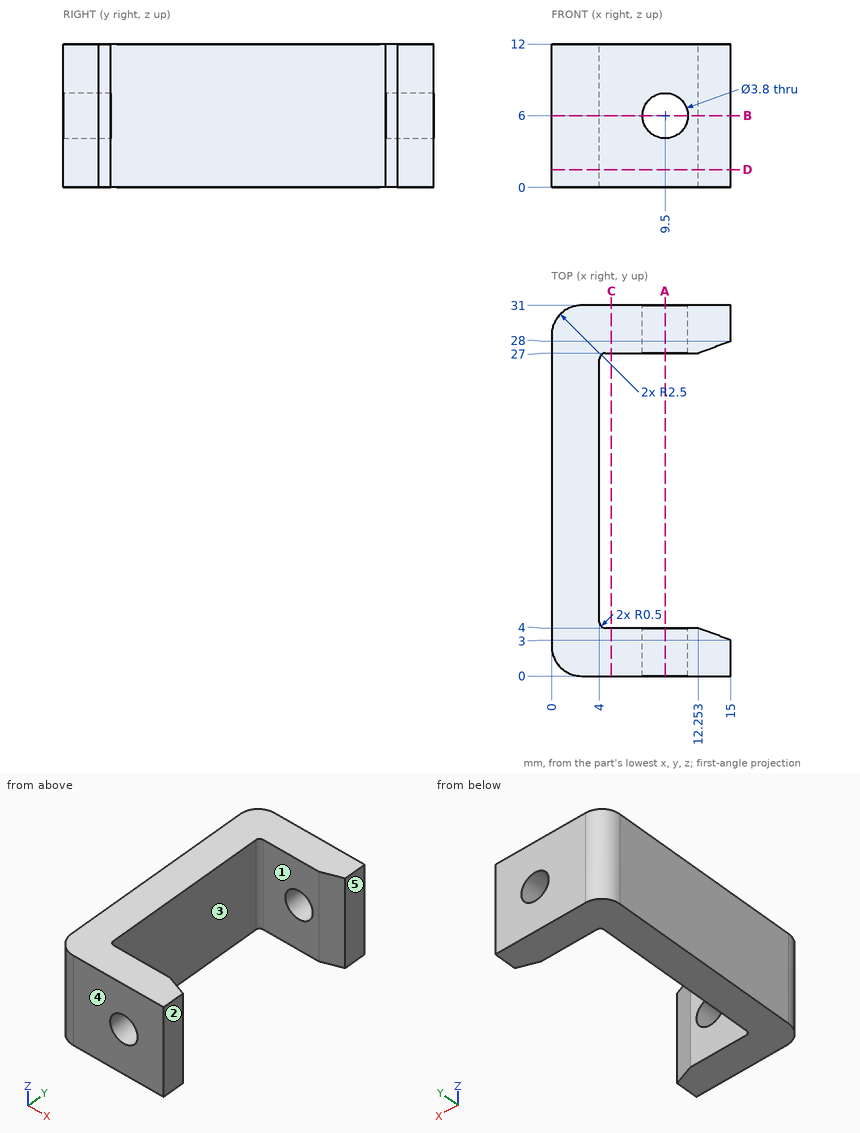
Check sheet for the drawn part. Datum: minimum x, y, z corner. Units: mm. A direction names the side the tool comes from. Round coordinates to 2 decimals unless told otherwise and drop trailing zeros. Order: outer loops, then holes, each group sorted by start corner. A loop starts at its lowest first (then second) coordinate and runs counter-clockwise, first axis right, second up. Notation, with made-up numbers: (10.5, 15) -> (38.5, 15) arc R37 cw to (38.5, 53) -> close; hole circle Ø9 at (53.5, -20). An arc over 180 degrees is marked (long way). Use CSV: the item, a comma, the result in double quotes.
(1) Cross-section at C-C (x = 5). Record the boundary of the cut face in (y, z).
Worked out:
outline,"(0, 0) -> (4, 0) -> (4, 12) -> (0, 12) -> close; (27, 0) -> (31, 0) -> (31, 12) -> (27, 12) -> close"
(2) Tool access check on the marked faces 1 and 2. Record the directions out of +Z, -Z, +X, -X, +Y, -Y that give a thin tool (end or side, any length) a straight path to the whole face; none if there is none.
Worked out:
face 1,"+Z, -Z, +X"
face 2,"+Z, -Z, +X, +Y, -Y"
(3) Depth check by flat-ended pin: pin 1 (2.5 mm diameter, centred on x = 9.5, z = 6, fed in from +Y); pin 2 (2 mm diameter, centred on y = 12, z = 7, fed in from +X). Enter the tip coordinate at first touch or a pass-through.
Worked out:
pin 1,"through"
pin 2,"x = 4"
(4) Cross-section at B-B (z = 6). Record the boundary of the cut face in (x, y), and give its area (3 significant figures).
Worked out:
outline,"(0, 2.5) arc R2.5 ccw to (2.5, 0) -> (7.6, 0) -> (7.6, 4) -> (4.5, 4) arc R0.5 cw to (4, 4.5) -> (4, 26.5) arc R0.5 cw to (4.5, 27) -> (7.6, 27) -> (7.6, 31) -> (2.5, 31) arc R2.5 ccw to (0, 28.5) -> close; (11.4, 0) -> (15, 0) -> (15, 3) -> (12.25, 4) -> (11.4, 4) -> close; (11.4, 27) -> (12.25, 27) -> (15, 28) -> (15, 31) -> (11.4, 31) -> close"
area,"176 mm²"
(5) Cross-section at D-D (z = 1.5). Record the boundary of the cut face in (x, y), and give its area (3 significant figures).
Worked out:
outline,"(0, 2.5) arc R2.5 ccw to (2.5, 0) -> (15, 0) -> (15, 3) -> (12.25, 4) -> (4.5, 4) arc R0.5 cw to (4, 4.5) -> (4, 26.5) arc R0.5 cw to (4.5, 27) -> (12.25, 27) -> (15, 28) -> (15, 31) -> (2.5, 31) arc R2.5 ccw to (0, 28.5) -> close"
area,"207 mm²"
(6) Cross-section at A-A (x = 9.5). Record the boundary of the cut face in (y, z).
Worked out:
outline,"(0, 0) -> (4, 0) -> (4, 4.1) -> (0, 4.1) -> close; (0, 7.9) -> (4, 7.9) -> (4, 12) -> (0, 12) -> close; (27, 0) -> (31, 0) -> (31, 4.1) -> (27, 4.1) -> close; (27, 7.9) -> (31, 7.9) -> (31, 12) -> (27, 12) -> close"
(7) Material ranges on line 1 along Y through (x, z) = (11.5, 11.75); line 2 along X through (y, z) = (25, 4.5); line 3 along X through (y, z) = (2.55, 6), recorded low to high. Write a range as from..to.
Worked out:
line 1,"0..4, 27..31"
line 2,"0..4"
line 3,"0..7.6, 11.4..15"
(8) Draft check along Y on the marked faces 3, 4 and 5. Enter one of: pulls with the +Y half, pulls with the -Y half, needs draft (parallel to the pull), parting line crosses it, or undercut.
Worked out:
face 3,"undercut"
face 4,"pulls with the -Y half"
face 5,"needs draft"
